Autodesk Inventor part; units mm, degrees
ref_plane "Work Plane1" through (1.525, 0, 0) normal (0, 0, 1) x (1, 0, 0)
ref_plane "YZ Plane" through (0, 0, 0) normal (1, 0, 0) x (0, 1, 0)
ref_plane "XZ Plane" through (0, 0, 0) normal (0, 1, 0) x (-1, 0, 0)
sketch "Sketch1" plane through (0, 0, 0) normal (0, 0, 1) x (1, 0, 0)
  line L0 (0, 9.5) -> (0, 6)
  line L1 (4, 6) -> (150, 6)
  line L2 (150, 6) -> (150, 0)
  line L3 (150, 0) -> (-0.4001, 0)
  line L4 (-30.4801, 0) -> (180.08, 0)
  line L5 (-0.4001, 0) -> (-0.4001, 9.5)
  line L6 (-0.4001, 9.5) -> (0, 9.5)
  line L7 (4, 6) -> (3.2331, 6)
  line L8 (3.2331, 6) -> (0, 6)
  line L9 (0, -1.9) -> (0, 11.4)
  dimension "d0" = 150
  dimension "d1" = 146
  dimension "d2" = 12
  dimension "d9" = 0.4001
  dimension "d10" = 19
  dimension "d13" = 0.7669
  dimension "d14" = 12
revolve "Body" add sketch "Sketch1" angle 360 about axis through (150, 0, 0) along (-1, 0, 0)
sketch "Sketch2" plane through (-0.4001, 0, 0) normal (-1, 0, 0) x (0, 0, 1)
  line L0 (0, 10.9697) -> (9.5, 5.4848)
  line L1 (9.5, 5.4848) -> (9.5, -5.4848)
  line L2 (9.5, -5.4848) -> (0, -10.9697)
  line L3 (0, -10.9697) -> (-9.5, -5.4848)
  line L4 (-9.5, -5.4848) -> (-9.5, 5.4848)
  line L5 (-9.5, 5.4848) -> (0, 10.9697)
  point P0 (0, 0)
  point P1 (0, 0)
  dimension "d11" = 19
extrude "Head" add sketch "Sketch2" along normal blind 7.6
sketch "Sketch4" plane through (0, 0, 0) normal (0, 0, 1) x (1, 0, 0)
  line L0 (-8.0001, 9.5) -> (-8.0001, 10.9697)
  line L1 (-8.0001, 10.9697) -> (-7.1516, 10.9697)
  line L2 (-7.1516, 10.9697) -> (-8.0001, 9.5)
  line L3 (-9.5201, 0) -> (1.1199, 0)
  line L4 (-0.4001, 10.9697) -> (-8.0001, 10.9697)
  line L5 (-8.0001, 5.4848) -> (-8.0001, 10.9697)
  dimension "d5" = 30
  dimension "d19" = 19
revolve "Chamfer1" cut sketch "Sketch4" angle 360 about axis through (-10, 0, 0) along (1, 0, 0)
thread "Thread"
chamfer "Chamfer2" distance 0.7668 distance2 0.7669 1 edges at (150, -6, 0) measured on face at (150, -1.326, -0.0818)
ref_plane "Work Plane1" through (1.525, 0, 0) normal (0, 0, 1) x (1, 0, 0)
equation "\"d0\" = NLG"
equation "\"d1\" = GEL"
equation "\"d2\" = GD"
equation "\"d10\" = SD2"
equation "\"d14\" = BDM"
equation "\"d11\" = SW"
equation "\"d3\" = KOH - SD"
equation "\"d5\" = ANG1"
equation "\"d19\" = SW0"
equation "\"d15\" = GEL"
equation "\"d6\" = -0.5 * SPD + 0.5 * GD"
equation "\"NLG\" = 150"
equation "\"GD\" = NND"
equation "\"BDM\" = NND"
equation "\"KOH\" = 8"
equation "\"GEL\" = 146"
equation "\"SW\" = 19"
equation "\"SW0\" = SW"
equation "\"SPD\" = NND - 1.2269 * PTC"
equation "\"SD2\" = SW"
equation "\"SD\" = WFT"
equation "\"ANG1\" = 30deg"
equation "\"GAL\" = 0.61345 * PTC"
equation "\"GUL\" = 0.61345 * PTC"
equation "\"RR\" = 0.6"
equation "\"WFT\" = 0.4"
equation "\"GD1\" = THREADDIA - 1.2269 * PTC"
equation "\"THREADDIA\" = 12"
equation "\"SDH\" = SW"
equation "\"TOA\" = 30deg"
equation "\"PTC\" = 1.25"
equation "\"NND\" = 12"
equation "\"E0\" = 1.155 * SW"
properties part number "CNS 4321 - M12 x 150" material "Steel, Mild"
Can you work these out from the model? Positions are in its coordinate system, mm. A direction names the side the tool comes from. Give positions to 0.01 mm unless a question says otherwise; leave off trailing zeros. Order: outer loops, then holes, each group sorted by start corner. A loop starts at its lowest first (then second) coordinate and runs counter-clockwise, first axis right, second up. Notation, with made-up numbers: M 7.25,-14 L 42.25,-14 A28 cw 42.25,23 Z; hole C 26.25,11.5 d1. An arc over 180 degrees is marked long. Use one line per item in the form item = value.
Item 1: For faces 1 (the flat face through (-0.4, -5, 9)), 2 (the flat face through (-0.4, 5, -9)), 3 (the flat face through (-0.4, -5, -9)), 4 (the cylindrical face through (74, -6, 0)), 5 (the flat face through (-0.4, -10, 0)), which set-ups out of +Z, -Z, +X, -X, +Y, -Y let a thin tool reach every point of the face, with its end or its side?
Values follow:
face_1 = +Z, +X, -Y
face_2 = -Z, +X, +Y
face_3 = -Z, +X, -Y
face_4 = +X
face_5 = +X, -Y
Item 2: If we section it at A-A, the plane x = 95.5: Write out the boundary of the cut face in (y, z).
Values follow:
outline = C 0,0 d12
Item 3: Will these pins go through, and if not, where does the flat tip stop? pin 1 Ø5 at (x, z) = (33.5, -4.5) entering from +Y; pin 2 Ø2.5 at (y, z) = (4, 6.5) entering from +X; pin 3 Ø10 at (x, z) = (71, 6.5) entering from -Y.
Values follow:
pin_1 = 5.66
pin_2 = 0
pin_3 = -5.81
Item 4: If I drill on line 1 along X through (y, z) = (-7, 3.25); line 2 along Y through (x, z) = (75.5, 0.25); line 3 along Z through (x, y) = (91, 2.75), over which ranges is the centre line in solid material (lowest first)? Write a range as [from, to].
Values follow:
line_1 = [-8, 0]
line_2 = [-5.99, 5.99]
line_3 = [-5.33, 5.33]
